Read the model definition and answer for the solid it produces. Units are mm, in the model's axes. Face numbers are marked on the shaded views. Round coordinates to 2 decimals unless told otherwise and drop trailing zeros. Write each loop counter-clockwise with the first axis right and the second up, starting at its lowest first coordinate (ties: lowest second). Pieces come first, ordered by that corner, then holes. Notation, with made-up numbers: (48, 52) -> (61, 52) arc R20 cw to (61, 59) -> close; hole circle Ø9 at (-21.75, 6). An arc over 180 degrees is marked (long way). Return JSON: item names as keys, results as strings. Group by question number.
(1) Given pin 1 (2 mm diameter, centred on x = 0.5, z = -1.5, fed in from +Y); pin 2 (4 mm diameter, centred on y = 0, z = 0, fed in from -X); pin 3 (2 mm diameter, centred on x = 2.5, z = -1.5, fed in from -Y), each flat-ended and moving along its own axis, determine where each tip first touches the part or whether it passes through.
(2) A cutting plane is placed at A-A on y = 0. Give the vertices of the cut face in (x, z), then the cut area to 3 significant figures.
(3) The mould has two halves that part along Y. Classify the marked faces 1, 2 and 3: released by +Y, released by -Y, zero draft, split by the parting line, or undercut.
(4) A cutting plane is placed at C-C on x = 3.3. Give the vertices of the cut face in (y, z).
(5) Straight lines are drawn through the part: line 1 (Y direction, x = 1.6, z = 0); line 2 (Y direction, x = 0.25, z = -1). For each, find the intervals that lie inside material, in ascending order.
```python
from build123d import *

# Parameters (mm, degrees)
FILLET1_R          = 0.2
FILLET2_R          = 0.2
HEX_2_DEPTH        = 2
SKETCH4_R          = 2.5
CUT_EXTRUDE1_DEPTH = 85.712469332
SKETCH9_R          = 2.5
CUT_EXTRUDE6_DEPTH = 353.231631037


with BuildPart() as part:
    # BodySke → Base-Revolve (revolve)
    with BuildSketch(Plane.XY, mode=Mode.PRIVATE) as base_revolve_sk:
        Polygon((0, 0), (0, 3.5), (4, 3.5), (4, 2), (15.61, 2), (16, 1.61), (16, 0), align=None)
    revolve(base_revolve_sk.sketch.rotate(Axis((-31.75, 0, 0), (1, 0, 0)), 90), axis=Axis((-31.75, 0, 0), (1, 0, 0)))

    # Fillet1
    fillet1_edges = [part.edges().sort_by_distance(p)[0] for p in [
        (4, 0, -2),
    ]]
    fillet(fillet1_edges, radius=FILLET1_R)

    # Fillet2
    fillet2_edges = [part.edges().sort_by_distance(p)[0] for p in [
        (0, 0, -3.5),
    ]]
    fillet(fillet2_edges, radius=FILLET2_R)

    # Sketch2 → Hex-PreBroach (revolve, cut)
    with BuildSketch(Plane.XY, mode=Mode.PRIVATE) as hex_prebroach_sk:
        Polygon((0, 1.5355), (2, 1.5355), (2.886521338, 0), (0, 0), align=None)
    revolve(hex_prebroach_sk.sketch.rotate(Axis((0, 0, 0), (1, 0, 0)), 90), axis=Axis((0, 0, 0), (1, 0, 0)), mode=Mode.SUBTRACT)

    # Sketch3 → Hex 2 (cut)
    with BuildSketch(Plane(origin=(0, 0, 0), x_dir=(0, 0.500000000000001, 0.866025403784438), z_dir=(-1, 0, 0))):
        Polygon((0.886521338, 1.5355), (-0.886521338, 1.5355), (-1.773042677, 0), (-0.886521338, -1.5355), (0.886521338, -1.5355), (1.773042677, 0), align=None)
    extrude(amount=-HEX_2_DEPTH, mode=Mode.SUBTRACT)

    # Sketch4 → Cut-Extrude1 (cut, through all)
    with BuildSketch(Plane(origin=(4, -67.297227621, -41.443909469), x_dir=(0, 0, 1), z_dir=(-1, 0, 0))):
        with Locations((41.443909469, 67.297227621)):
            Circle(SKETCH4_R)
    extrude(amount=-CUT_EXTRUDE1_DEPTH, mode=Mode.SUBTRACT)

    # Sketch9 → Cut-Extrude6 (cut, through all)
    with BuildSketch(Plane(origin=(254, -186.360303269, -149.810753298), x_dir=(0, 0.9242245927363031, 0.3818493186865921), z_dir=(1, 0, 0))):
        with Locations(Location((229.443909469, 67.297227621, 0), (0, 0, 337.551719153))):
            Circle(SKETCH9_R)
    extrude(amount=-CUT_EXTRUDE6_DEPTH, mode=Mode.SUBTRACT)


solid = part.part
```
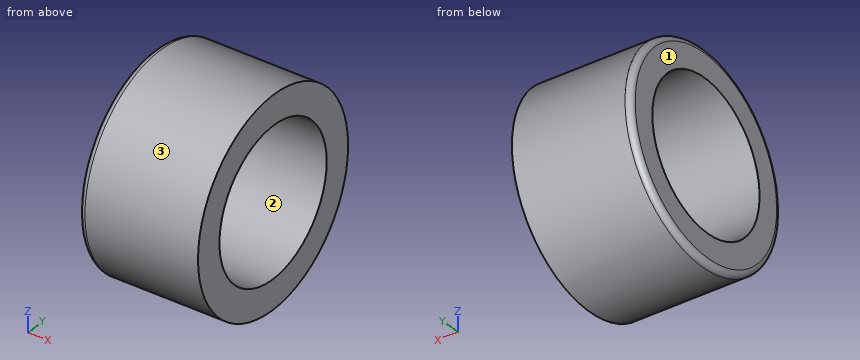
Checks:
{
 "1": {"pin 1": "stops at y = 3.46", "pin 2": "passes through", "pin 3": "stops at y = -3.46"},
 "2": {"outline": "(0, -3.3) arc R0.2 ccw to (0.2, -3.5) -> (4, -3.5) -> (4, -2.5) -> (0, -2.5) -> close; (0, 2.5) -> (4, 2.5) -> (4, 3.5) -> (0.2, 3.5) arc R0.2 ccw to (0, 3.3) -> close", "area": "7.98 mm^2"},
 "3": {"face 1": "zero draft", "face 2": "undercut", "face 3": "split by the parting line"},
 "4": {"outline": "circle Ø7 at (0, 0); hole circle Ø5 at (0, 0)"},
 "5": {"line 1": "y = -3.5 to -2.5, 2.5 to 3.5", "line 2": "y = -3.35 to -2.29, 2.29 to 3.35"}
}
